Could you check a few things on this model? Use its own coordinates, in mm. Face numbers are marked on the shaded views. A direction names the side the tool comes from. Coordinates: 2 decimals unless noted, no trailing zeros. Order: outer loops, then holes, each group sorted by start corner. A loop starts at its lowest first (then second) coordinate and runs counter-clockwise, first axis right, second up. Notation, with made-up numbers: (-35.75, 71.5) - (-20.75, 71.5) arc R17 ccw to (-20.75, 76.5) - close; hole circle Ø4 at (-6, -27). An arc over 180 degrees is marked (long way). Answer as a JSON object with one key per item and string values. Group by question number.
(1) Imagine slicing it at B-B, the plane x = 109.5. Write out the boundary of the cut face in (y, z), and give its area (3 significant figures).
(2) Will this pin go through, and if not, where does the flat tip stop? P1, Ø4.5, axis at x = 142, z = 55, coming from the +Y side.
(3) Imagine slicing it at C-C, the plane z = 25. Write out the boundary of the cut face in (x, y), and give its area (3 significant figures).
(4) Imagine slicing it at A-A, the plane y = 21. Write out the boundary of the cut face in (x, z).
(5) We'd pull the mould along Z, two halves only. Please class the marked faces 1, 2 and 3: pulls with the +Z half, pulls with the -Z half, needs draft (parallel to the pull), parting line crosses it, or undercut.
(6) Which directions (+Z, -Z, +X, -X, +Y, -Y) give clear straight access to the entire face, cutting with the end or side of a thin tool? Please do the marked faces 4 and 5.
(7) Please list where these lines run through material, in increasing order: probe 1 along Z at (x, y) = (130, 45.5); probe 2 along X at (y, z) = (45.25, 55); probe 3 along X at (y, z) = (6, -15.5).
from build123d import *

# Parameters (mm, degrees)
BOSS_EXTRUDE1_DEPTH       = 50
SHELL1_T                  = -1
BOSS_EXTRUDE3_START       = 5
BOSS_EXTRUDE3_DEPTH       = 1
F_5_0MM_DOWEL_HOLE2_D     = 5
F_5_0MM_DOWEL_HOLE2_DEPTH = 1
F_5_0MM_DOWEL_HOLE3_D     = 5
F_5_0MM_DOWEL_HOLE3_DEPTH = 1


with BuildPart() as part:
    # Sketch1 → Boss-Extrude1 (new body)
    with BuildSketch(Plane(origin=(0, 0, 0), x_dir=(1, 0, 0), z_dir=(0, 1, 0))):
        with BuildLine():
            Line((-130, -75), (130, -75))
            ThreePointArc((130, -75), (144.142135624, -69.142135624), (150, -55))
            Line((150, -55), (150, 55))
            ThreePointArc((150, 55), (144.142135624, 69.142135624), (130, 75))
            Line((130, 75), (-130, 75))
            ThreePointArc((-130, 75), (-144.142135624, 69.142135624), (-150, 55))
            Line((-150, 55), (-150, -55))
            ThreePointArc((-150, -55), (-144.142135624, -69.142135624), (-130, -75))
        make_face()
    extrude(amount=BOSS_EXTRUDE1_DEPTH)

    # Shell1
    shell1_openings = [part.faces().sort_by_distance(p)[0] for p in [
        (0, 50, 0),
    ]]
    offset(amount=SHELL1_T, openings=shell1_openings, kind=Kind.INTERSECTION)

    # Sketch3 → Boss-Extrude3 (add)
    with BuildSketch(Plane(origin=(0, 50, 0), x_dir=(-1, 0, 0), z_dir=(0, -1, 0)).offset(BOSS_EXTRUDE3_START)):
        with BuildLine():
            Line((130, 75), (-130, 75))
            ThreePointArc((-130, 75), (-144.142135624, 69.142135624), (-150, 55))
            Line((-150, 55), (-150, -55))
            ThreePointArc((-150, -55), (-144.142135624, -69.142135624), (-130, -75))
            Line((-130, -75), (130, -75))
            ThreePointArc((130, -75), (144.142135624, -69.142135624), (150, -55))
            Line((150, -55), (150, 55))
            ThreePointArc((150, 55), (144.142135624, 69.142135624), (130, 75))
        make_face()
        with BuildLine():
            Line((130, -60), (-130, -60))
            ThreePointArc((-130, -60), (-133.535533906, -58.535533906), (-135, -55))
            Line((-135, -55), (-135, 55))
            ThreePointArc((-135, 55), (-133.535533906, 58.535533906), (-130, 60))
            Line((-130, 60), (130, 60))
            ThreePointArc((130, 60), (133.535533906, 58.535533906), (135, 55))
            Line((135, 55), (135, -55))
            ThreePointArc((135, -55), (133.535533906, -58.535533906), (130, -60))
        make_face(mode=Mode.SUBTRACT)
    extrude(amount=-BOSS_EXTRUDE3_DEPTH)

    # Ø5.0mm Dowel Hole2
    with Locations(Plane(origin=(0, 46, 0), x_dir=(1, 0, 0), z_dir=(0, 1, 0))):
        with Locations((-65, 67), (65, 67), (142, 0), (-142, 0), (-65, -67), (65, -67)):
            Hole(F_5_0MM_DOWEL_HOLE2_D / 2, depth=F_5_0MM_DOWEL_HOLE2_DEPTH)

    # Ø5.0mm Dowel Hole3
    with Locations(Plane(origin=(0, 46, 0), x_dir=(1, 0, 0), z_dir=(0, 1, 0))):
        with Locations((-130, 67), (-142, 55), (-142, -55), (-130, -67), (130, -67), (142, -55), (142, 55), (130, 67)):
            Hole(F_5_0MM_DOWEL_HOLE3_D / 2, depth=F_5_0MM_DOWEL_HOLE3_DEPTH)


solid = part.part
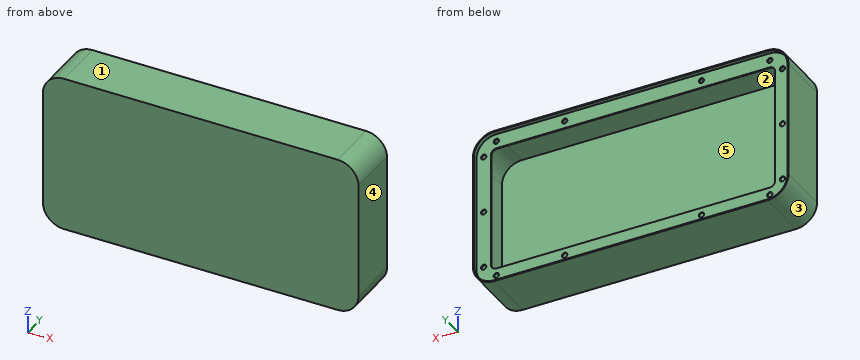
Result set:
{
 "1": {"outline": "(0, -75) - (50, -75) - (50, -74) - (46, -74) - (46, -60) - (45, -60) - (45, -74) - (1, -74) - (1, 74) - (45, 74) - (45, 60) - (46, 60) - (46, 74) - (50, 74) - (50, 75) - (0, 75) - close", "area": "276 mm^2"},
 "2": {"P1": "stops at y = 1"},
 "3": {"outline": "(-150, 0) - (150, 0) - (150, 50) - (149, 50) - (149, 46) - (135, 46) - (135, 45) - (149, 45) - (149, 1) - (-149, 1) - (-149, 45) - (-135, 45) - (-135, 46) - (-149, 46) - (-149, 50) - (-150, 50) - close", "area": "426 mm^2"},
 "4": {"outline": "(-150, -55) arc R20 ccw to (-130, -75) - (130, -75) arc R20 ccw to (150, -55) - (150, 55) arc R20 ccw to (130, 75) - (-130, 75) arc R20 ccw to (-150, 55) - close; hole (-149, -55) arc R19 ccw to (-130, -74) - (130, -74) arc R19 ccw to (149, -55) - (149, 55) arc R19 ccw to (130, 74) - (-130, 74) arc R19 ccw to (-149, 55) - close"},
 "5": {"face 1": "pulls with the +Z half", "face 2": "undercut", "face 3": "pulls with the -Z half"},
 "6": {"face 4": "+Z, -Z, +X, +Y, -Y", "face 5": "none"},
 "7": {"probe 1": "z = -75 to -69.5, -64.5 to -60, 60 to 64.5, 69.5 to 75", "probe 2": "x = -150 to -144.5, -139.5 to -135, 135 to 139.5, 144.5 to 150", "probe 3": "x = -150 to -149, 149 to 150"}
}
